Source: CAD feature listing. Evaluate the final solid. Frame: model axes, mm. A direction names the side the tool comes from. Coordinates: 2 decimals unless noted, no trailing zeros. Loops run counter-clockwise (first coordinate to the right, second up) from the corner with the lowest first, then second, coordinate; pieces in that order, holes last. Notation, with made-up numbers: (68, 0.25) -> (76, 0.25) arc R28 cw to (76, 38.25) -> close; hole circle Ø7 at (-28, 5.25). An arc over 180 degrees is marked (long way). Answer as CSV lines item,"result".
from build123d import *

# Parameters (mm, degrees)
SKETCH1_W           = 200
SKETCH1_H           = 200
BOSS_EXTRUDE1_DEPTH = 71
FILLET1_R           = 20
SKETCH2_R           = 10
BOSS_EXTRUDE2_DEPTH = 30


with BuildPart() as part:
    # Sketch1 → Boss-Extrude1 (new body)
    with BuildSketch(Plane(origin=(0, 0, 0), x_dir=(1, 0, 0), z_dir=(0, 1, 0))):
        Rectangle(SKETCH1_W, SKETCH1_H)
    extrude(amount=BOSS_EXTRUDE1_DEPTH)

    # Fillet1
    fillet1_edges = [part.edges().sort_by_distance(p)[0] for p in [
        (100, 35.5, 100),
        (-100, 35.5, 100),
        (-100, 35.5, -100),
        (100, 35.5, -100),
    ]]
    fillet(fillet1_edges, radius=FILLET1_R)

    # Sketch2 → Boss-Extrude2 (add)
    with BuildSketch(Plane.XY.offset(100)):
        with Locations(Location((-30, 12, 0), (0, 0, 180))):
            Circle(SKETCH2_R)
    extrude(amount=BOSS_EXTRUDE2_DEPTH)


solid = part.part
(1) Cut plane D-D (z = 103). Return the cut outline in (x, y), then the cut area to 3 significant figures.
Computed values:
outline,"circle Ø20 at (-30, 12)"
area,"314 mm^2"
(2) Pin query (flat end, axial travel): pin 1 Ø4 at (x, y) = (53, 59.5) entering from +Z. Return the tip coordinate at first contact, or that it passes through.
Computed values:
pin 1,"z = 100"
(3) Cut plane C-C (y = 54). Return the cut outline in (x, z).
Computed values:
outline,"(-100, -80) arc R20 ccw to (-80, -100) -> (80, -100) arc R20 ccw to (100, -80) -> (100, 80) arc R20 ccw to (80, 100) -> (-80, 100) arc R20 ccw to (-100, 80) -> close"
(4) Access query for faces 1 (the cylindrical face through (-39.54, 9, 114.79)), 2 (the cylindrical face through (93.986, 35.997, 94.297)). Directions: +Z, -Z, +X, -X, +Y, -Y. A direction counts if a zero-diameter tool reaches every point of the face in a straight line with its end or side. Return the directions, or none.
Computed values:
face 1,"+Z"
face 2,"+Z, +X, +Y, -Y"
(5) Cut plane B-B (x = -30). Return the cut outline in (y, z).
Computed values:
outline,"(0, -100) -> (71, -100) -> (71, 100) -> (22, 100) -> (22, 130) -> (2, 130) -> (2, 100) -> (0, 100) -> close"
(6) Material intervals for L1, parallel to Z at x = -56, y = 34; L2, parallel to X at y = 32.5, z = 85.5; L3, parallel to X at y = 5.5, z = 114, sorted ascending. Write a range as [from, to].
Computed values:
L1,"[-100, 100]"
L2,"[-99.23, 99.23]"
L3,"[-37.6, -22.4]"
(7) Cut plane A-A (y = 12). Return the cut outline in (x, z), then the cut area to 3 significant figures.
Computed values:
outline,"(-100, -80) arc R20 ccw to (-80, -100) -> (80, -100) arc R20 ccw to (100, -80) -> (100, 80) arc R20 ccw to (80, 100) -> (-20, 100) -> (-20, 130) -> (-40, 130) -> (-40, 100) -> (-80, 100) arc R20 ccw to (-100, 80) -> close"
area,"40,300 mm^2"
